Design review of the part built by this model. Coordinates are the model's own, in mm. A direction names the side the tool comes from. Give positions to 0.01 mm unless a question says otherwise; leave off trailing zeros. Loops run counter-clockwise (first coordinate to the right, second up) from the corner with the lowest first, then second, coordinate; pieces in that order, holes last. Notation, with made-up numbers: M 37,0 L 61,0 A20 cw 61,34 Z; hole C 5,-37.75 d3. An arc over 180 degrees is marked long. Answer as CSV lines item,"result".
Autodesk Fusion 360 part; units mm, degrees
sketch "Sketch1" plane through (0, 0, 0) normal (0, 0, 1) x (1, 0, 0)
  line L0 (0, 0) -> (20, 0)
  line L1 (20, 40) -> (0, 40)
  line L2 (0, 40) -> (0, 0)
  circle A0 centre (20, 20) radius 10
  arc A1 (20, 0) -> (20, 40) centre (20, 20) ccw
  dimension "d1" = 20
  dimension "d2" = 40
  dimension "d3" = 20
  dimension "d10" = 20
sketch "Sketch2" plane through (0, 0, 0) normal (1, 0, 0) x (0, 1, 0)
  line L0 (0, 0) -> (40, 0)
  line L1 (40, 0) -> (40, 50.06)
  line L2 (40, 50.06) -> (0, 50.06)
  line L3 (0, 50.06) -> (0, 0)
  dimension "d4" = 40
  dimension "d5" = 50.06
ref_plane "WorkPlane1" through (20, 20, 50.06) normal (0, 0, 1) x (1, 0, 0)
sketch "Sketch3" plane through (20, 20, 50.06) normal (0, 0, 1) x (1, 0, 0)
  line L0 (-20, 20) -> (-5, 20)
  line L1 (0, 15) -> (0, -15)
  line L2 (-5, -20) -> (-20, -20)
  line L3 (-20, -20) -> (-20, 20)
  arc A0 (-5, -20) -> (0, -15) centre (-5, -15) ccw
  arc A1 (0, 15) -> (-5, 20) centre (-5, 15) ccw
  point P0 (0, 20)
  dimension "d7" = 20
  dimension "d8" = 40
  dimension "d9" = 5
extrude "Extrude1" add sketch "Sketch1" along normal blind 10
extrude "Extrude2" add sketch "Sketch2" against normal blind 10
extrude "Extrude3" add sketch "Sketch3" against normal blind 10
fillet "Fillet1" radius 10 1 edges at (0, 20, 10)
fillet "Fillet2" radius 10 1 edges at (-10, 20, 0)
1. The part is to be moulded in two halves that separate along Z. For faces 4 (the flat face through (-2, 40, 25)), 5 (the flat face through (10, 20, 40.06)), 6 (the cylindrical face through (-6.99, 20.28, 2.85)), say which applies: pulls with the +Z half, pulls with the -Z half, needs draft (parallel to the pull), parting line crosses it, or undercut.
Answer block:
face 4,"needs draft"
face 5,"undercut"
face 6,"pulls with the -Z half"
2. To check wall thickness, follow L1, parallel to Y at x = 20, z = 3; L2, parallel to Z at x = 19, y = 31; L3, parallel to Z at x = 1, y = 13.5. State the ranges of each line that lie inside material, in increasing order. Write a range as [from, to].
Answer block:
L1,"[0, 10], [30, 40]"
L2,"[0, 10], [40.06, 50.06]"
L3,"[0, 15.64], [40.06, 50.06]"
3. For faces 1 (the cylindrical face through (19, 38, 45)), 2 (the cylindrical face through (18, 1, 45)), 3 (the flat face through (31, 20, 10)), list the 3-axis set-ups (+Z, -Z, +X, -X, +Y, -Y) from which the entire face can be reached by the end or side of a thin tool; tool diameter is ignored.
Answer block:
face 1,"+Z, +X, +Y"
face 2,"+Z, +X, -Y"
face 3,"+X, +Y, -Y"
4. We need section D-D, the plane y = 37.5. Write out the cut boundary in (x, z), plus the area to 3 significant figures.
Answer block:
outline,"M -10,10 A10 ccw 0,0 L 29.68,0 L 29.68,10 L 10,10 A10 cw 0,20 L 0,40.06 L 19.33,40.06 L 19.33,50.06 L -10,50.06 Z"
area,"991 mm²"
5. We need section C-C, the plane z = 5.5. Write out the cut boundary in (x, y).
Answer block:
outline,"M -8.93,0 L 20,0 A20 ccw 20,40 L -8.93,40 Z; hole C 20,20 d20"
6. We need section B-B, the plane x = 5. Write out the cut boundary in (y, z), plus the area to 3 significant figures.
Answer block:
outline,"M 0,0 L 40,0 L 40,11.34 L 0,11.34 Z; M 0,40.06 L 40,40.06 L 40,50.06 L 0,50.06 Z"
area,"854 mm²"
7. We need section A-A, the plane y = 24. Write out the cut boundary in (x, z), plus the area to 3 significant figures.
Answer block:
outline,"M -10,10 A10 ccw 0,0 L 10.83,0 L 10.83,10 L 10,10 A10 cw 0,20 L 0,40.06 L 20,40.06 L 20,50.06 L -10,50.06 Z; M 29.17,0 L 39.6,0 L 39.6,10 L 29.17,10 Z"
area,"913 mm²"
8. For P1, Ø9, axis at x = 27, y = 29, coming from the +Z side; P2, Ø3, axis at y = 23.5, z = 43.5, coming from the +X side; P3, Ø8, axis at x = 33.5, z = 9.5, coming from the +Y side, all flat-tipped, find the tip position at first contact; note any pin that passes through.
Answer block:
P1,"z = 10"
P2,"x = 20"
P3,"y = 37.6"
